```python
from build123d import *

# Parameters (mm, degrees)
F3_ANGLE_BACK = 15
F3_ANGLE      = 30
F4_ANGLE_BACK = 13
F4_ANGLE      = 26
F5_ANGLE      = 15


# Not quite as in the source:
# - a feature of the source that left no trace in its solid (it failed there, or was rolled back) is left out


with BuildPart() as f3:
    # F0 (on Right) → F3 (revolve)
    with BuildSketch(Plane.YZ, mode=Mode.PRIVATE) as f3_sk:
        Polygon((-198.3431457505, -4), (-196, -1.6568542495), (-196, -0.2), (-204, -0.2), (-204, -1.6568542495), (-201.6568542495, -4), align=None)
    revolve(f3_sk.sketch.rotate(Axis((0, 0, 14.9391144514), (0, 0, -1)), -F3_ANGLE_BACK), axis=Axis((0, 0, 14.9391144514), (0, 0, -1)), revolution_arc=F3_ANGLE)

    # F2 (on Right) → F4 (revolve)
    with BuildSketch(Plane.YZ, mode=Mode.PRIVATE) as f4_sk:
        Polygon((-195, 1.6568542495), (-197.3431457505, 4), (-202.6568542495, 4), (-205, 1.6568542495), (-205, -1.6568542495), (-202.6568542495, -4), (-197.3431457505, -4), (-195, -1.6568542495), align=None)
    revolve(f4_sk.sketch.rotate(Axis((0, 0, 27.1144676954), (0, 0, 1)), -F4_ANGLE_BACK), axis=Axis((0, 0, 27.1144676954), (0, 0, 1)), revolution_arc=F4_ANGLE)


with BuildPart() as f3_1:
    # F5: moved
    add(f3.part.rotate(Axis((0, 0, 14.9391144514), (0, 0, -1)), F5_ANGLE))


solid = f3_1.part
```
Design review of the part built by this model. Coordinates are the model's own, in mm. A direction names the side the tool comes from. Coordinates: 2 decimals unless noted, no trailing zeros. Write each loop counter-clockwise with the first axis right and the second up, starting at its lowest first coordinate (ties: lowest second). Pieces come first, ordered by that corner, then holes. Notation, with made-up numbers: M -30.75,8 L 6.25,8 A13 cw 6.25,29 Z; hole C 57,70 d3. An arc over 180 degrees is marked long. Answer as a JSON object with one key per item and string values.
Item 1: Add section B-B, the plane z = 2.75. Give the boundary of the cut face in (x, y), and give its area (3 significant figures).
Outcome:
{"outline": "M -95.73,-180.04 A203.91 ccw -7.12,-203.78 L -6.84,-195.97 A196.09 cw -92.06,-173.14 Z", "area": "709 mm²"}
Item 2: Insertion check: pin 1 Ø2 at (x, y) = (-4, -200) entering from +Z; pin 2 Ø2 at (x, z) = (-70.5, -2) entering from -Y. Each pin has a flat end and moves straight along its axis. Give the tip position at first contact, or say it passes through.
Outcome:
{"pin 1": "z = -0.2", "pin 2": "y = -192.84"}
Item 3: Add section A-A, the plane z = -3. Give the boundary of the cut face in (x, y), and give its area (3 significant figures).
Outcome:
{"outline": "M -101.33,-175.51 A202.66 ccw -95.14,-178.94 L -95.61,-179.82 A203.66 ccw -7.11,-203.53 L -7.07,-202.53 A202.66 ccw 0,-202.66 L 0,-197.34 A197.34 cw -6.89,-197.22 L -6.85,-196.22 A196.34 cw -92.18,-173.36 L -92.65,-174.24 A197.34 cw -98.67,-170.9 Z", "area": "738 mm²"}
Item 4: Machinability: for faces 1 (the flat face through (-97, -175, -0.2)), 2 (the conical face through (-3.49, -202.782, -2.845)), 3 (the conical face through (-95.54, -172.46, -2.81)), 4 (the conical face through (-53.17, -195.94, -3.63)), 5 (the conical face through (-51.166, -188.555, -2.031)), which of the approach directions +Z, -Z, +X, -X, +Y, -Y give a long, thin tool a straight path to every point of the face, cutting with its end or side? Answer none if there is none.
Outcome:
{"face 1": "+Z, -X, +Y", "face 2": "-Z, -Y", "face 3": "-Z, +Y", "face 4": "-Z, -X, -Y", "face 5": "-Z, +X, +Y"}
Item 5: Draft analysis for pull direction X (two halves, no side actions). For faces 6 (the cylindrical face through (-94.98, -171.45, -0.92)), 7 (the flat face through (-51, -191, 4)), 8 (the conical face through (-51.174, -188.587, 2.064)), state which applies: pulls with the +X half, pulls with the -X half, needs draft (parallel to the pull), parting line crosses it, or undercut.
Outcome:
{"face 6": "undercut", "face 7": "needs draft", "face 8": "pulls with the +X half"}
Item 6: Wall thickness on probe 1 along Y at (x, z) = (-88.5, 1); probe 2 along X at (y, z) = (-177, 1.75); probe 3 along Y at (x, z) = (-36, 1): over which ranges is each line inside the solid? List them lowest first.
Outcome:
{"probe 1": "-184.91 to -173.76", "probe 2": "-94.11 to -82.05", "probe 3": "-201.81 to -191.65"}
